Autodesk Inventor part; units mm, degrees
ref_plane "YZ Plane" through (0, 0, 0) normal (1, 0, 0) x (0, 1, 0)
ref_plane "XZ Plane" through (0, 0, 0) normal (0, 1, 0) x (-1, 0, 0)
ref_plane "XY Plane" through (0, 0, 0) normal (0, 0, 1) x (1, 0, 0)
sketch "Sketch1" plane through (0, 0, 0) normal (0, 1, 0) x (-1, 0, 0)
  line L0 (0, 0) -> (15, 0)
  line L1 (15, 0) -> (15, -29.5)
  line L2 (15, -29.5) -> (0, -29.5)
  line L3 (0, -29.5) -> (0, 0)
  dimension "d0" = 15
  dimension "d1" = 29.5
extrude "Extrusion1" add sketch "Sketch1" along normal blind 5
fillet "Fillet1" radius 5 2 edges at (-7.5, 5, 0) (-7.5, 5, -29.5)
fillet "Fillet2" radius 4.074 1 edges at (0, 0, -14.75)
sketch "Sketch2" plane through (0, 0, 0) normal (0, -1, 0) x (1, 0, 0)
  circle A0 centre (-3.581, -10) radius 1.5
  line L0 (-15, -29.5) -> (-15, 0)
  line L1 (-15, -14.75) -> (-4.074, -14.75)
  line L2 (-4.074, 0) -> (-4.074, -29.5)
  circle A1 centre (-3.581, -19.5) radius 1.5
  line L3 (0, -27.3987) -> (0, -2.1013)
  point P0 (0, 0)
  dimension "d6" = 3
  dimension "d7" = 4.75
  dimension "d8" = 10.926
  dimension "d10" = 3
  dimension "d11" = 4.75
  dimension "d15" = 3.581
  dimension "d16" = 3.581
extrude "Extrusion2" cut sketch "Sketch2" against normal up to surface (5 mm away)
fillet "Fillet3" radius 1.993 1 edges at (-15, 0, -14.75)
sketch "Sketch3" plane through (0, 0, 0) normal (0, -1, 0) x (1, 0, 0)
  circle A0 centre (-3.581, -10) radius 2.5
  circle A1 centre (-3.581, -19.5) radius 2.5
  circle A2 centre (-3.581, -10) radius 1.5
  circle A3 centre (-3.581, -19.5) radius 1.5
  point P0 (0, 0)
  dimension "d18" = 5
  dimension "d19" = 5
  dimension "d20" = 0
  dimension "d21" = 0
  dimension "d22" = 0
  dimension "d23" = 0
extrude "Extrusion3" cut sketch "Sketch3" against normal blind 0.75
properties part number "bottomclip" material "ABS Plastic"
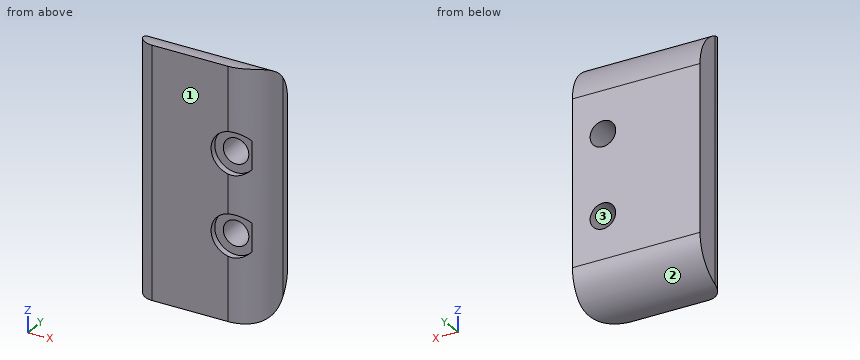
Verification items for the finished model (mm, model axes). Face numbers are marked on the shaded views. Coordinates: 2 decimals unless noted, no trailing zeros. Write each loop counter-clockwise with the first axis right and the second up, starting at its lowest first coordinate (ties: lowest second). Pieces come first, ordered by that corner, then holes. Notation, with made-up numbers: M 86.5,-37 L 131.5,-37 A27 cw 131.5,0 Z; hole C -16,61.25 d6. An arc over 180 degrees is marked long. One line per question, with ' | ' between items.
1) Sectioned sample at C-C on y = 2.7. Record the cut outline in (x, z), then the cut area to 3 significant figures.
Solutions:
outline: M -15,-28.71 L -0.24,-28.71 L -0.24,-0.79 L -15,-0.79 Z; hole C -3.58,-19.5 d3; hole C -3.58,-10 d3 | area: 398 mm^2
2) Depth check by flat-ended pin: pin 1 Ø4.5 at (x, z) = (-3.581, -10) entering from -Y; pin 2 Ø3 at (x, y) = (-10.5, 4) entering from +Z; pin 3 Ø5 at (x, z) = (-3, -10) entering from -Y. Enter the tip coordinate at first touch or a pass-through.
Solutions:
pin 1: y = 0.75 | pin 2: z = -0.67 | pin 3: y = 0.08
3) Sectioned sample at B-B on x = -2.5. Record the cut outline in (y, z), then the cut area to 3 significant figures.
Solutions:
outline: M 0.32,-29.49 A5 ccw 5,-24.5 L 5,-20.54 L 0.75,-20.54 L 0.75,-21.75 L 0.32,-21.75 Z; M 0.32,-17.25 L 0.75,-17.25 L 0.75,-18.46 L 5,-18.46 L 5,-11.04 L 0.75,-11.04 L 0.75,-12.25 L 0.32,-12.25 Z; M 0.32,-7.75 L 0.75,-7.75 L 0.75,-8.96 L 5,-8.96 L 5,-5 A5 ccw 0.32,-0.01 Z | area: 106 mm^2
4) Sectioned sample at A-A on z = -19.5. Record the cut outline in (x, y), then the cut area to 3 significant figures.
Solutions:
outline: M -15,1.99 A1.99 ccw -13.01,0 L -6.08,0 L -6.08,0.75 L -5.08,0.75 L -5.08,5 L -15,5 Z; M -2.08,0.75 L -1.72,0.75 A4.07 ccw 0,4.07 L 0,5 L -2.08,5 Z | area: 55.1 mm^2
5) Material ranges on L1, parallel to Z at x = -3.75, y = 2.7; L2, parallel to Z at x = -4.25, y = 3.85; L3, parallel to X at y = 2.3, z = -11.25, recorded low to high.
Solutions:
L1: -28.71 to -20.99, -18.01 to -11.49, -8.51 to -0.79 | L2: -27.69 to -20.84, -18.16 to -11.34, -8.66 to -1.81 | L3: -15 to -4.41, -2.75 to -0.41
6) Release check for a two-part mould opening along Z. For the marked faces 1, 2 and 3 record: +Z half, -Z half, draft (parallel to the pull), parting line (faces both ways), or undercut.
Solutions:
face 1: draft | face 2: -Z half | face 3: undercut
